Check sheet for the modelled part. Datum: model origin and axes. Units: mm. Face numbers are marked on the shaded views. A direction names the side the tool comes from. Give positions to 0.01 mm unless a question says otherwise; leave off trailing zeros. Loops run counter-clockwise (first coordinate to the right, second up) from the corner with the lowest first, then second, coordinate; pieces in that order, holes last. Notation, with made-up numbers: (7.5, -40) - (41.5, -40) arc R8 ccw to (41.5, -33) - close; hole circle Ø11 at (23.5, 5.5). An arc over 180 degrees is marked (long way). Use CSV: the item, a comma, the result in double quotes.
from build123d import *

# Parameters (mm, degrees)
SKETCH008_R     = 2.1
PAD003_DEPTH    = 10
POCKET005_DEPTH = 3
SKETCH010_R     = 3.5
POCKET006_DEPTH = 3.5


with BuildPart() as part:
    # Sketch008 → Pad003 (new body)
    with BuildSketch(Plane.XY):
        with BuildLine():
            Line((7.31364, 0.727262), (5.35154, 9))
            ThreePointArc((5.35154, 9), (0, 13.23074), (-5.35154, 9))
            Line((-5.35154, 9), (-7.31364, 0.727262))
            ThreePointArc((-8, 0), (-7.559385, 0.271676), (-7.31364, 0.727262))
            Line((-14, 0), (-8, 0))
            ThreePointArc((-14.86632, 0.499489), (-14.500079, 0.133679), (-14, 0))
            Line((-20.638485, 10.483552), (-14.86632, 0.499489))
            ThreePointArc((-20.638485, 10.483552), (-29.007959, 11.88196), (-28.789459, 3.399278))
            Line((-15.5, -7), (-28.789459, 3.399278))
            Line((-15.5, -0.5), (-15.5, -7))
            Line((8, -0.5), (-15.5, -0.5))
            Line((8, 0), (8, -0.5))
            ThreePointArc((7.31364, 0.727262), (7.559385, 0.271676), (8, 0))
        make_face()
        with Locations((-25.4, 7.73074)):
            Circle(SKETCH008_R, mode=Mode.SUBTRACT)
        with Locations((0, 7.73074)):
            Circle(SKETCH008_R, mode=Mode.SUBTRACT)
    extrude(amount=PAD003_DEPTH)

    # Sketch009 (on Face5 of Pad003) → Pocket005 (cut)
    with BuildSketch(Plane(origin=(0, 0, 0), x_dir=(-1, 0, 0), z_dir=(0, 1, 0))):
        Polygon((12.365, 2.801443), (13.49, 4.75), (12.365, 6.698557), (10.115, 6.698557), (8.99, 4.75), (10.115, 2.801443), align=None)
    extrude(amount=-POCKET005_DEPTH, mode=Mode.SUBTRACT)

    # Sketch010 (on Face5 of Pocket005) → Pocket006 (cut)
    with BuildSketch(Plane.XY.offset(10)):
        with Locations((-25.4, 7.73074)):
            Circle(SKETCH010_R)
        with Locations((0, 7.73074)):
            Circle(SKETCH010_R)
    extrude(amount=-POCKET006_DEPTH, mode=Mode.SUBTRACT)


solid = part.part
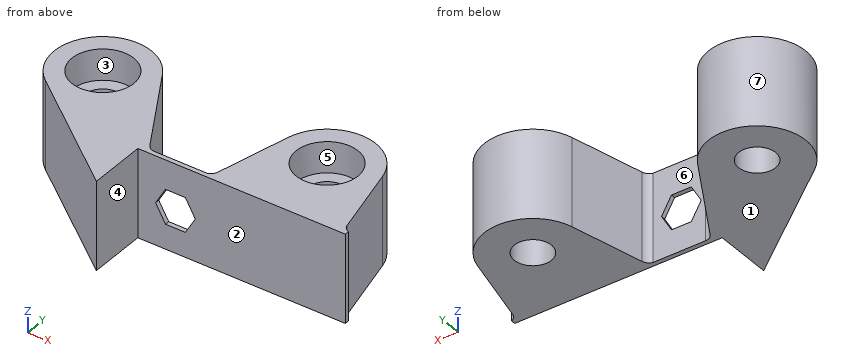
1. Go/stop test with flat-tipped pins: pin 1 Ø1.5 at (x, z) = (-3.5, 2) entering from -Y; pin 2 Ø2 at (y, z) = (-3.5, 3) entering from +X; pin 3 Ø4 at (y, z) = (2.5, 7.5) entering from -X. Record where each tip stops, or that it passes through.
Completed:
pin 1,"stops at y = -0.5"
pin 2,"stops at x = -15.5"
pin 3,"stops at x = -29.85"
2. Release check for a two-part mould opening along Y. For the marked faces 1, 2 and 3 record: released by +Y, released by -Y, zero draft, split by the parting line, or undercut.
Completed:
face 1,"zero draft"
face 2,"released by -Y"
face 3,"undercut"
3. Set-up check for the marked faces 4, 5, 6 and 7: record each of +Z, -Z, +X, -X, +Y, -Y from which the full face is reachable in a straight line by a thin tool's end or side.
Completed:
face 4,"+Z, -Z, +X, -Y"
face 5,"+Z"
face 6,"+Z, -Z, +Y"
face 7,"+Z, -Z"
4. Scan lines: line 1 along X through (y, z) = (7, 7.25); line 2 along X through (y, z) = (8, 7.75); line 3 along Y through (x, z) = (-25.4, 8.6). Record each from-to range of solid material in increasing order.
Completed:
line 1,"x = -30.85 to -28.82, -21.98 to -18.62, -5.83 to -3.42, 3.42 to 5.83"
line 2,"x = -30.89 to -28.89, -21.91 to -19.2, -5.59 to -3.49, 3.49 to 5.59"
line 3,"y = 0.75 to 4.23, 11.23 to 13.23"
5. Sectioned sample at B-B, the plane z = 6. Record the boundary of the cut face in (x, y).
Completed:
outline,"(-28.79, 3.4) - (-15.5, -7) - (-15.5, -0.5) - (-12.77, -0.5) - (-12.77, 0) - (-14, 0) arc R1 cw to (-14.87, 0.5) - (-20.64, 10.48) arc R5.5 ccw (long way) to start; (-9.71, -0.5) - (8, -0.5) - (8, 0) arc R1 cw to (7.31, 0.73) - (5.35, 9) arc R5.5 ccw to (-5.35, 9) - (-7.31, 0.73) arc R1 cw to (-8, 0) - (-9.71, 0) - close; hole circle Ø4.2 at (-25.4, 7.73); hole circle Ø4.2 at (0, 7.73)"
6. Sectioned sample at C-C, the plane y = 2.5. Record the boundary of the cut face in (x, z), and give its area (3 significant figures).
Completed:
outline,"(-27.64, 0) - (-16.02, 0) - (-16.02, 10) - (-27.64, 10) - close; (-6.89, 0) - (6.89, 0) - (6.89, 10) - (-6.89, 10) - close"
area,"254 mm²"
7. Sectioned sample at A-A, the plane x = 0. Record the boundary of the cut face in (y, z).
Completed:
outline,"(-0.5, 0) - (5.63, 0) - (5.63, 6.5) - (4.23, 6.5) - (4.23, 10) - (-0.5, 10) - close; (9.83, 0) - (13.23, 0) - (13.23, 10) - (11.23, 10) - (11.23, 6.5) - (9.83, 6.5) - close"
8. Sectioned sample at D-D, the plane x = -25.4. Record the boundary of the cut face in (y, z), and give its area (3 significant figures).
Completed:
outline,"(0.75, 0) - (5.63, 0) - (5.63, 6.5) - (4.23, 6.5) - (4.23, 10) - (0.75, 10) - close; (9.83, 0) - (13.23, 0) - (13.23, 10) - (11.23, 10) - (11.23, 6.5) - (9.83, 6.5) - close"
area,"73.0 mm²"
